from build123d import *

# Parameters (mm, degrees)
F1_R     = 11
F1_W     = 7.2
F1_H     = 4.2
F2_DEPTH = 1
F0_R     = 5.65
F0_R_2   = 5.15
F3_DEPTH = 4.5
F4_R     = 1


with BuildPart() as f2:
    # F1 (on Top) → F2 (new body)
    with BuildSketch(Plane.XY):
        Circle(F1_R)
        Rectangle(F1_W, F1_H, mode=Mode.SUBTRACT)
    extrude(amount=F2_DEPTH)

    # F0 (on Top) → F3 (join)
    with BuildSketch(Plane.XY):
        Circle(F0_R)
        Circle(F0_R_2, mode=Mode.SUBTRACT)
    extrude(amount=F3_DEPTH)

    # F4
    f4_edges = [f2.edges().sort_by_distance(p)[0] for p in [
        (-5.65, 0, 1),
    ]]
    fillet(f4_edges, radius=F4_R)


solid = f2.part
Here's how the part is built. I have some questions about the finished solid (model axes, mm). A direction names the side the tool comes from. Coordinates: 2 decimals unless noted, no trailing zeros. Loops run counter-clockwise (first coordinate to the right, second up) from the corner with the lowest first, then second, coordinate; pieces in that order, holes last. Notation, with made-up numbers: (74.5, 62) -> (81.5, 62) arc R13 cw to (81.5, 67) -> close; hole circle Ø5 at (3, 15). An arc over 180 degrees is marked (long way). Use one line per item in the form item = value. Start each with the question number.
(1) On a 3-axis mill with a long thin cutter (end or side, diameter ignored), from which of +Z, -Z, +X, -X, +Y, -Y can I reach the whole of each face in a straight line? I mean faces 1 (the face through (-0.1, -2.1, 0.5)), 2 (the face through (4.91, 1.55, 2.73)), 3 (the face through (-0.2, -2.3, 0)). Say none if no direction works.
(2) If we section it at C-C (z = 1.4): Please give me the cut outline in (x, y), then the cut area to 3 significant figures.
(3) Will these pins go through, and if not, where does the flat tip stop? pin 1 (4 mm diameter, centred on x = 2, y = 8, fed in from +Z); pin 2 (0.5 mm diameter, centred on y = -1, z = 0.5, fed in from -X); pin 3 (2 mm diameter, centred on x = -4.5, z = 3, fed in from -Y).
(4) If we section it at A-A (x = 0): Please give me the cut outline in (y, z), then the cut area to 3 significant figures.
(5) If we section it at D-D (z = 4.1): Please give me the cut outline in (x, y).
(6) We'd pull the mould along X, two halves only. Please class faces 4 (the face through (3.6, 0, 0.5)), 5 (the face through (-2.38, -10.74, 0.49)), 6 (the face through (5, -5, 1)): pulls with the +X half, pulls with the -X half, needs draft (parallel to the pull), parting line crosses it, or undercut.
(7) Please list where these lines run through material, in increasing order: line 1 along X through (y, z) = (0, 3.2); line 2 along X through (y, z) = (0, 1.75).
(8) If we section it at B-B (y = 0): Please give me the cut outline in (x, z), then the cut area to 3 significant figures.
Verdict:
q1.face_1 = +Z, -Z
q1.face_2 = +Z
q1.face_3 = -Z, +X, -X, +Y, -Y
q2.outline = circle Ø11.7 at (0, 0); hole circle Ø10.3 at (0, 0)
q2.area = 24.2 mm²
q3.pin_1 = 1.09
q3.pin_2 = -10.97
q3.pin_3 = -4.44
q4.outline = (-11, 0) -> (-2.1, 0) -> (-2.1, 1) -> (-5.15, 1) -> (-5.15, 4.5) -> (-5.65, 4.5) -> (-5.65, 2) arc R1 cw to (-6.65, 1) -> (-11, 1) -> close; (2.1, 0) -> (11, 0) -> (11, 1) -> (6.65, 1) arc R1 cw to (5.65, 2) -> (5.65, 4.5) -> (5.15, 4.5) -> (5.15, 1) -> (2.1, 1) -> close
q4.area = 21.7 mm²
q5.outline = circle Ø11.3 at (0, 0); hole circle Ø10.3 at (0, 0)
q6.face_4 = undercut
q6.face_5 = parting line crosses it
q6.face_6 = needs draft
q7.line_1 = -5.65 to -5.15, 5.15 to 5.65
q7.line_2 = -5.68 to -5.15, 5.15 to 5.68
q8.outline = (-11, 0) -> (-3.6, 0) -> (-3.6, 1) -> (-5.15, 1) -> (-5.15, 4.5) -> (-5.65, 4.5) -> (-5.65, 2) arc R1 cw to (-6.65, 1) -> (-11, 1) -> close; (3.6, 0) -> (11, 0) -> (11, 1) -> (6.65, 1) arc R1 cw to (5.65, 2) -> (5.65, 4.5) -> (5.15, 4.5) -> (5.15, 1) -> (3.6, 1) -> close
q8.area = 18.7 mm²
